Source: CAD feature listing. Evaluate the final solid. Frame: model axes, mm. A direction names the side the tool comes from. Round coordinates to 2 decimals unless told otherwise and drop trailing zeros. Write each loop counter-clockwise with the first axis right and the second up, starting at its lowest first coordinate (ties: lowest second). Pieces come first, ordered by that corner, then holes. Notation, with made-up numbers: (57.25, 44.25) - (98.25, 44.25) arc R23 cw to (98.25, 67.25) - close; hole circle Ø3 at (88, 58.5). An arc over 180 degrees is marked (long way). Write item = value, one per line. Start each with the question number.
```python
from build123d import *

# Parameters (mm, degrees)
F0_R     = 10
F0_R_2   = 4.5
F0_R_3   = 3.25
F1_DEPTH = 3
F2_DEPTH = 35
F3_R     = 1


with BuildPart() as f1:
    # F0 (on Top) → F1 (new body)
    with BuildSketch(Plane.XY):
        Circle(F0_R)
        Circle(F0_R_2, mode=Mode.SUBTRACT)
        Circle(F0_R_2)
        Circle(F0_R_3, mode=Mode.SUBTRACT)
    extrude(amount=F1_DEPTH)

    # F0 (on Top) → F2 (join)
    with BuildSketch(Plane.XY):
        Circle(F0_R_2)
        Circle(F0_R_3, mode=Mode.SUBTRACT)
    extrude(amount=F2_DEPTH)

    # F3
    f3_edges = [f1.edges().sort_by_distance(p)[0] for p in [
        (-4.5, 0, 35),
        (-3.25, 0, 0),
    ]]
    fillet(f3_edges, radius=F3_R)


solid = f1.part
```
(1) Section D-D (y = 6). Return the cut outline in (x, z).
(2) Section A-A (x = 0). Return the cut outline in (y, z), plus the area to 3 significant figures.
(3) Contact query for flat-ended pins moving along their axis: P1, Ø5, axis at x = -4.5, z = 23, coming from the +Y side; P2, Ø3, axis at x = 0.5, y = 7, coming from the +Z side; P3, Ø8, axis at x = -6.5, z = 22.5, coming from the -Y side. Output: stop coordinate, or through.
(4) Pull-direction query (X, two-part tool) for faces 1 (the cylindrical face through (-2.579, -1.978, 17.762)), 2 (the cylindrical face through (-2.17, -9.76, 1.48)), 3 (the flat face through (4.3, -2.1, 3)); classes: +X half, -X half, draft (parallel to the pull), parting line (faces both ways), or undercut.
(5) Reachability of faces 4 (the flat face through (2, -4, 0)), 5 (the cylindrical face through (-0.59, 4.46, 18.28)) from +Z, -Z, +X, -X, +Y, -Y: full face, straight path, thin tool, end or side. Return the list, or none.
(6) Section C-C (z = 20.5). Return the cut outline in (x, y), plus the area to 3 significant figures.
(7) Ray query, L1, parallel to Y at x = 0, z = 14; L2, parallel to Z at x = -6.5, y = 4.25; L3, parallel to Y at x = 3, z = 7. Return the intervals inside material, ascending. Write a range as from..to.
Solution:
q1.outline = (-8, 0) - (8, 0) - (8, 3) - (-8, 3) - close
q2.outline = (-10, 0) - (-4.25, 0) arc R1 ccw to (-3.25, 1) - (-3.25, 35) - (-3.5, 35) arc R1 ccw to (-4.5, 34) - (-4.5, 3) - (-10, 3) - close; (3.25, 1) arc R1 ccw to (4.25, 0) - (10, 0) - (10, 3) - (4.5, 3) - (4.5, 34) arc R1 ccw to (3.5, 35) - (3.25, 35) - close
q2.area = 120 mm^2
q3.P1 = 4.03
q3.P2 = 3
q3.P3 = -3.74
q4.face_1 = undercut
q4.face_2 = parting line
q4.face_3 = draft
q5.face_4 = -Z, +X, -X, +Y, -Y
q5.face_5 = +Z
q6.outline = circle Ø9 at (0, 0); hole circle Ø6.5 at (0, 0)
q6.area = 30.4 mm^2
q7.L1 = -4.5..-3.25, 3.25..4.5
q7.L2 = 0..3
q7.L3 = -3.35..-1.25, 1.25..3.35
